```python
from build123d import *

# Parameters (mm, degrees)
F1_DEPTH = 76.2
F2_R     = 12.7
F3_DEPTH = 76.201
F5_DEPTH = 25.4
F8_DEPTH = 6.35
F9_R     = 38.1
F10_R    = 38.1
F11_SIZE = 15.24


# Not quite as in the source:
# - a pattern or mirror of a feature is missing from the dataset's text; its kind, count and spacing are read off the source's solid


with BuildPart() as f1:
    # F0 (on Top) → F1 (new body, symmetric)
    with BuildSketch(Plane.XY):
        Polygon((-76.2, 25.4), (-76.2, 0), (0, 0), (0, 152.4), (-25.4, 152.4), (-25.4, 25.4), align=None)
    extrude(amount=F1_DEPTH, both=True)

    # F2 (on face) → F3 (cut, through all)
    with BuildSketch(Plane.YZ):
        with Locations((114.3, 0)):
            Circle(F2_R)
    extrude(amount=-F3_DEPTH, mode=Mode.SUBTRACT)

    # F4 (on face) → F5 (cut)
    with BuildSketch(Plane.XZ):
        with BuildLine():
            ThreePointArc((-63.5, -12.7), (-50.8, 0), (-63.5, 12.7))
            Line((-63.5, 12.7), (-76.2, 12.7))
            Line((-76.2, 12.7), (-76.2, -12.7))
            Line((-76.2, -12.7), (-63.5, -12.7))
        make_face()
    extrude(amount=-F5_DEPTH, mode=Mode.SUBTRACT)

    # F7 (on offset) → F8 (join, symmetric)
    with BuildSketch(Plane.XY.offset(44.45)):
        Polygon((-50.8, 25.4), (-25.4, 25.4), (-25.4, 109.758593142), align=None)
    f8 = extrude(amount=F8_DEPTH, both=True)

    # F8_copies: F8 across plane
    add(f8.mirror(Plane(origin=(0, 0, 0), x_dir=(-1, 0, 0), z_dir=(0, 0, -1))))

    # F9
    f9_edges = [f1.edges().sort_by_distance(p)[0] for p in [
        (-12.7, 152.4, 76.2),
    ]]
    fillet(f9_edges, radius=F9_R)

    # F10
    f10_edges = [f1.edges().sort_by_distance(p)[0] for p in [
        (-12.7, 152.4, -76.2),
    ]]
    fillet(f10_edges, radius=F10_R)

    # F11
    f11_edges = [f1.edges().sort_by_distance(p)[0] for p in [
        (-25.4, 101.6, 0),
    ]]
    chamfer(f11_edges, length=F11_SIZE)


solid = f1.part
```
Check sheet for the modelled part. Datum: model origin and axes. Units: mm. A direction names the side the tool comes from. Coordinates: 2 decimals unless noted, no trailing zeros. Write each loop counter-clockwise with the first axis right and the second up, starting at its lowest first coordinate (ties: lowest second). Pieces come first, ordered by that corner, then holes. Notation, with made-up numbers: (87.25, 86) -> (110.25, 86) arc R15 cw to (110.25, 102) -> close; hole circle Ø10 at (77, 46). An arc over 180 degrees is marked (long way). Use a Markdown table: item, result.
1. Go/stop test with flat-tipped pins: pin 1 Ø15 at (y, z) = (114.3, 0) entering from -X; pin 2 Ø8 at (x, z) = (-29.5, -60.5) entering from +Y; pin 3 Ø12.5 at (x, y) = (-32.5, 88.5) entering from +Z; pin 4 Ø4 at (y, z) = (133, 6) entering from -X. Record where each tip stops, or that it passes through.
Reported:
| item | result |
|---|---|
| pin 1 | passes through |
| pin 2 | stops at y = 25.4 |
| pin 3 | stops at z = 50.8 |
| pin 4 | stops at x = -19.1 |
2. Sectioned sample at C-C (x = -53). Enter the section's corners in (y, z).
Reported:
| item | result |
|---|---|
| outline | (0, -76.2) -> (25.4, -76.2) -> (25.4, -7.14) -> (0, -7.14) -> close; (0, 7.14) -> (25.4, 7.14) -> (25.4, 76.2) -> (0, 76.2) -> close |
3. Sectioned sample at A-A (z = 0). Enter the section's corners in (x, y), plus the area to 3 significant figures.
Reported:
| item | result |
|---|---|
| outline | (-50.8, 0) -> (0, 0) -> (0, 101.6) -> (-10.16, 101.6) -> (-25.4, 86.36) -> (-25.4, 25.4) -> (-50.8, 25.4) -> close; (-25.4, 142.24) -> (-10.16, 127) -> (0, 127) -> (0, 152.4) -> (-25.4, 152.4) -> close |
| area | 3,640 mm2 |
4. Tool access check on faces 4 (the flat face through (-33, 49, -50.8)), 5 (the flat face through (-39, 0, 1)), 6 (the flat face through (-50, 25.4, 1)), 7 (the flat face through (-22, 45, -76.2)), 8 (the flat face through (-70, 13, -12.7)). Record the directions out of +Z, -Z, +X, -X, +Y, -Y that give a thin tool (end or side, any length) a straight path to the whole face; none if there is none.
Reported:
| item | result |
|---|---|
| face 4 | -Z, -X, +Y |
| face 5 | +Z, -Z, +X, -X, -Y |
| face 6 | -X, +Y |
| face 7 | -Z, +X, -X, +Y, -Y |
| face 8 | -X, +Y, -Y |
5. Sectioned sample at B-B (x = -22.5). Enter the section's corners in (y, z).
Reported:
| item | result |
|---|---|
| outline | (0, -76.2) -> (114.3, -76.2) arc R38.1 ccw to (152.4, -38.1) -> (152.4, 38.1) arc R38.1 ccw to (114.3, 76.2) -> (0, 76.2) -> close; hole circle Ø50.08 at (114.3, 0) |
6. Sectioned sample at D-D (y = 69). Enter the section's corners in (x, z), plus the area to 3 significant figures.
Reported:
| item | result |
|---|---|
| outline | (-37.67, -50.8) -> (-25.4, -50.8) -> (-25.4, -76.2) -> (0, -76.2) -> (0, 76.2) -> (-25.4, 76.2) -> (-25.4, 50.8) -> (-37.67, 50.8) -> (-37.67, 38.1) -> (-25.4, 38.1) -> (-25.4, -38.1) -> (-37.67, -38.1) -> close |
| area | 4,180 mm2 |
7. Scan lines: line 1 along Z through (x, y) = (-72, 19); line 2 along Z through (x, y) = (-27, 65.5); line 3 along Y through (x, z) = (-72.5, 20). Record each from-to range of solid material in increasing order.
Reported:
| item | result |
|---|---|
| line 1 | z = -76.2 to -12.7, 12.7 to 76.2 |
| line 2 | z = -50.8 to -38.1, 38.1 to 50.8 |
| line 3 | y = 0 to 25.4 |
8. Release check for a two-part mould opening along Z. For faces 1 (the flat face through (-33, 49, -38.1)), 2 (the cylindrical face through (-12.88, 141.54, -64.74)), 3 (the cylindrical face through (-12.88, 140.94, 65.34)) record: pulls with the +Z half, pulls with the -Z half, needs draft (parallel to the pull), parting line crosses it, or undercut.
Reported:
| item | result |
|---|---|
| face 1 | undercut |
| face 2 | pulls with the -Z half |
| face 3 | pulls with the +Z half |
